Check sheet for the drawn part. Datum: minimum x, y, z corner. Units: mm. Coordinates: 2 decimals unless noted, no trailing zeros. Loops run counter-clockwise (first coordinate to the right, second up) from the corner with the lowest first, then second, coordinate; pieces in that order, holes last. Notation, with made-up numbers: M 54.5,35.5 L 96.5,35.5 A19 cw 96.5,51.5 Z; hole C 4.25,79 d6. An arc over 180 degrees is marked long. Answer as CSV lines item,"result". Start each with the question number.
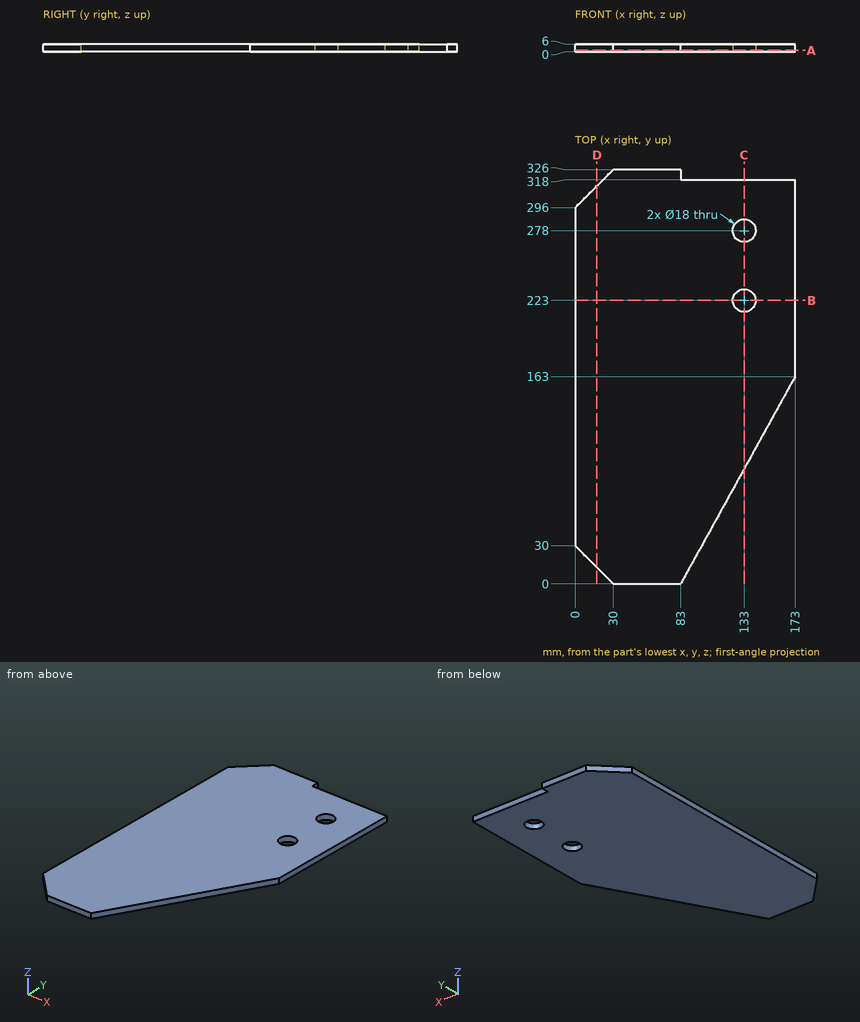
Item 1: Sectioned sample at C-C, the plane x = 133. Record the boundary of the cut face in (y, z), and give its area (3 significant figures).
Item 2: Material ranges on line 1 (X direction, y = 223, z = 4.4); line 2 (Y direction, x = 133, z = 3.95); line 3 (X direction, y = 224.5, z = 2.5), recorded low to high. Write a range as from..to.
Item 3: Sectioned sample at D-D, the plane x = 17. Record the boundary of the cut face in (y, z).
Item 4: Go/stop test with flat-tipped pins: pin 1 (14.5 mm diameter, centred on x = 133, y = 278, fed in from -Z); pin 2 (23.5 mm diameter, centred on x = 133, y = 223, fed in from -Z). Record where each tip stops, or that it passes through.
Item 5: Sectioned sample at A-A, the plane z = 0.9. Record the boundary of the cut face in (x, y), and give its area (3 significant figures).
Item 6: Sectioned sample at B-B, the plane y = 223. Record the boundary of the cut face in (x, z).
Reply:
1,outline,"M 90.56,0 L 214,0 L 214,6 L 90.56,6 Z; M 232,0 L 269,0 L 269,6 L 232,6 Z; M 287,0 L 318,0 L 318,6 L 287,6 Z"
1,area,"1,150 mm²"
2,line 1,"0..124, 142..173"
2,line 2,"90.56..214, 232..269, 287..318"
2,line 3,"0..124.13, 141.87..173"
3,outline,"M 13,0 L 313,0 L 313,6 L 13,6 Z"
4,pin 1,"through"
4,pin 2,"z = 0"
5,outline,"M 0,30 L 30,0 L 83,0 L 173,163 L 173,318 L 83,318 L 83,326 L 30,326 L 0,296 Z; hole C 133,223 d18; hole C 133,278 d18"
5,area,"46,900 mm²"
6,outline,"M 0,0 L 124,0 L 124,6 L 0,6 Z; M 142,0 L 173,0 L 173,6 L 142,6 Z"
